Input: part model. Units: mm. Frame: model coordinates. Round coordinates to 2 decimals unless told otherwise and drop trailing zeros. Order: outer loops, then holes, each group sorted by start corner. A loop starts at its lowest first (then second) coordinate and runs counter-clockwise, first axis right, second up. Notation, with made-up numbers: M -21,64.5 L 19,64.5 A19 cw 19,87.5 Z; hole C -24.5,73.5 d6. An arc over 180 degrees is marked long. One line per question, with ' | ' between items.
```python
from build123d import *

# Parameters (mm, degrees)
F0_R     = 10.9982
F1_DEPTH = 7.112
F2_R     = 3.1242


with BuildPart() as f1:
    # F0 (on Top) → F1 (new body)
    with BuildSketch(Plane.XY):
        with BuildLine():
            ThreePointArc((5.256284, 18.310488), (0, 13.178931), (-5.256284, 18.310488))
            ThreePointArc((-5.256284, 18.310488), (-13.470691, 13.470078), (-18.310727, 5.255451))
            ThreePointArc((-18.310727, 5.255451), (-13.17977, 0), (-18.310727, -5.255451))
            ThreePointArc((-18.310727, -5.255451), (-13.470691, -13.470078), (-5.256284, -18.310488))
            ThreePointArc((-5.256284, -18.310488), (0, -13.178933), (5.256284, -18.310488))
            ThreePointArc((5.256284, -18.310488), (13.47069, -13.470078), (18.310727, -5.255452))
            ThreePointArc((18.310727, -5.255452), (13.179773, 0), (18.310727, 5.255452))
            ThreePointArc((18.310727, 5.255452), (13.47069, 13.470078), (5.256284, 18.310488))
        make_face()
        Circle(F0_R, mode=Mode.SUBTRACT)
    extrude(amount=F1_DEPTH)

    # F2
    f2_edges = [f1.edges().sort_by_distance(p)[0] for p in [
        (-13.470691, 13.470078, 7.112),
        (-13.470691, -13.470078, 7.112),
        (13.47069, -13.470078, 7.112),
        (13.47069, 13.470078, 7.112),
        (13.47069, 13.470078, 0),
        (-13.470691, 13.470078, 0),
        (-13.470691, -13.470078, 0),
        (13.47069, -13.470078, 0),
    ]]
    fillet(f2_edges, radius=F2_R)


solid = f1.part
```
Item 1: Section query D-D, the plane z = 5.25. Return loops of the section in (x, y), plus the area to 3 significant figures.
Report:
outline: M -18.04,-5.24 A18.78 ccw -5.24,-18.04 A5.26 cw 5.24,-18.04 A18.78 ccw 18.04,-5.24 A5.26 cw 18.04,5.24 A18.78 ccw 5.24,18.04 A5.26 cw -5.24,18.04 A18.78 ccw -18.04,5.24 A5.26 cw Z; hole C 0,0 d22 | area: 551 mm²
Item 2: Mould query, pull axis Y, two halves, no side actions, for faces 1 (the cylindrical face through (-13.18, 0.11, 3.51)), 2 (the cylindrical face through (0.11, 13.18, 3.51)), 3 (the flat face through (-7, 10, 0)). Classes: +Y half, -Y half, draft (parallel to the pull), parting line (faces both ways), or undercut.
Report:
face 1: undercut | face 2: +Y half | face 3: draft
Item 3: First-contact query: pin 1 (2 mm diameter, centred on y = 7.5, z = 1.5, fed in from -X). Flat tip, straight axial feed; report the tip coordinate or a pass-through.
Report:
pin 1: x = -17.65
Item 4: Line query: line 1 along Y through (x, z) = (0, 4.5); line 2 along X through (y, z) = (15.5, 1.25); line 3 along Y through (x, z) = (-7, 6). Output: solid intervals per line, ascending. Write a range as from..to.
Report:
line 1: -13.18..-11, 11..13.18 | line 2: -9.96..-4.36, 4.36..9.96 | line 3: -16.93..-8.48, 8.48..16.93
Item 5: Section query A-A, the plane y = 0. Return loops of the section in (x, z), plus the area to 3 significant figures.
Report:
outline: M -13.18,0 L -11,0 L -11,7.11 L -13.18,7.11 Z; M 11,0 L 13.18,0 L 13.18,7.11 L 11,7.11 Z | area: 31.0 mm²
Item 6: Section query C-C, the plane z = 2. Return loops of the section in (x, y), plus the area to 3 significant figures.
Report:
outline: M -18.1,-5.25 A18.84 ccw -5.25,-18.1 A5.26 cw 5.25,-18.1 A18.84 ccw 18.1,-5.25 A5.26 cw 18.1,5.25 A18.84 ccw 5.25,18.1 A5.26 cw -5.25,18.1 A18.84 ccw -18.1,5.25 A5.26 cw Z; hole C 0,0 d22 | area: 555 mm²
